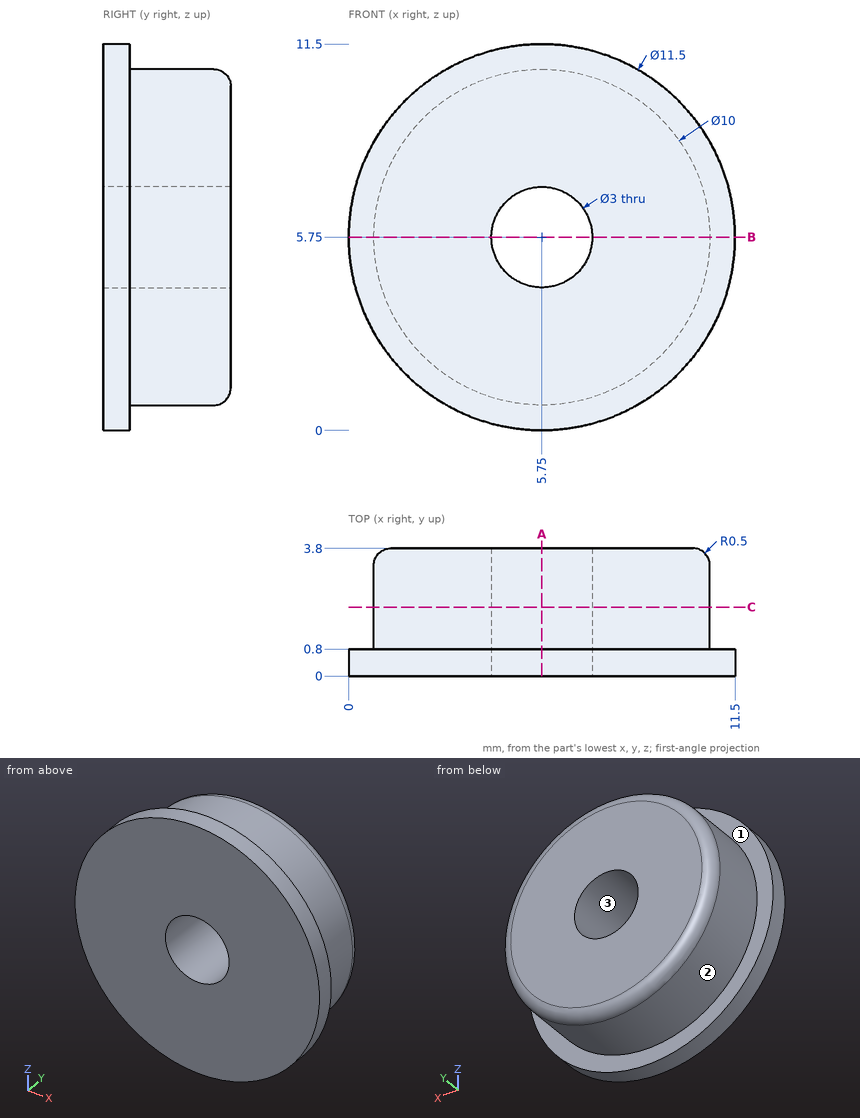
Source: three-view drawing plus pictorial views. Frame: mm from the lowest corner of the part. Coordinates: 2 decimals unless noted, no trailing zeros. Loops run counter-clockwise (first coordinate to the right, second up) from the corner with the lowest first, then second, coordinate; pieces in that order, holes last. Notation, with made-up numbers: (-12.75, 73.5) - (30.25, 73.5) arc R17 cw to (30.25, 89.5) - close; hole circle Ø10 at (25.5, 33.25). An arc over 180 degrees is marked (long way). Answer in a Markdown table with one row per item. Add a question column.
Item 1: Section query C-C on y = 2.05. Return the cut outline in (x, z).
Item 2: Contact query for flat-ended pins moving along their axis: P1, Ø2, axis at y = 0.5, z = 7.5, coming from the +X side; P2, Ø2.5, axis at x = 5.75, z = 5.75, coming from the +Y side. Output: stop coordinate, or through.
Item 3: Section query B-B on z = 5.75. Return the cut outline in (x, y), then the cut area to 3 significant figures.
Item 4: Line query: line 1 along X through (y, z) = (2.5, 5.75); line 2 along Z through (x, y) = (6.25, 1.75); line 3 along Z through (x, y) = (1.25, 0.5). Output: solid intervals per line, ascending. Write a range as [from, to].
Item 5: Mould query, pull axis X, two halves, no side actions, for the marked faces 1, 2 and 3. Classes: released by +X, released by -X, zero draft, split by the parting line, or undercut.
Item 6: Section query A-A on x = 5.75. Return the cut outline in (y, z).
Recorded:
| question | item | result |
|---|---|---|
| 1 | outline | circle Ø10 at (5.75, 5.75); hole circle Ø3 at (5.75, 5.75) |
| 2 | P1 | x = 11.45 |
| 2 | P2 | through |
| 3 | outline | (0, 0) - (4.25, 0) - (4.25, 3.8) - (1.25, 3.8) arc R0.5 ccw to (0.75, 3.3) - (0.75, 0.8) - (0, 0.8) - close; (7.25, 0) - (11.5, 0) - (11.5, 0.8) - (10.75, 0.8) - (10.75, 3.3) arc R0.5 ccw to (10.25, 3.8) - (7.25, 3.8) - close |
| 3 | area | 27.7 mm^2 |
| 4 | line 1 | [0.75, 4.25], [7.25, 10.75] |
| 4 | line 2 | [0.78, 4.34], [7.16, 10.72] |
| 4 | line 3 | [2.17, 9.33] |
| 5 | face 1 | zero draft |
| 5 | face 2 | split by the parting line |
| 5 | face 3 | undercut |
| 6 | outline | (0, 0) - (0.8, 0) - (0.8, 0.75) - (3.3, 0.75) arc R0.5 ccw to (3.8, 1.25) - (3.8, 4.25) - (0, 4.25) - close; (0, 7.25) - (3.8, 7.25) - (3.8, 10.25) arc R0.5 ccw to (3.3, 10.75) - (0.8, 10.75) - (0.8, 11.5) - (0, 11.5) - close |
